Autodesk Inventor part; units mm, degrees
ref_plane "YZ Plane" through (0, 0, 0) normal (1, 0, 0) x (0, 1, 0)
ref_plane "XZ Plane" through (0, 0, 0) normal (0, 1, 0) x (-1, 0, 0)
ref_plane "XY Plane" through (0, 0, 0) normal (0, 0, 1) x (1, 0, 0)
sketch "Sketch1" plane through (0, 0, 0) normal (0, 1, 0) x (-1, 0, 0)
  line L0 (-25, -25) -> (25, -25)
  line L1 (25, -25) -> (25, 25)
  line L2 (25, 25) -> (-25, 25)
  line L3 (-25, 25) -> (-25, -25)
  line L4 (-25, -25) -> (25, 25) construction
  line L5 (25, -25) -> (-25, 25) construction
  point P0 (0, 0)
  dimension "d0" = 50
  dimension "d1" = 50
extrude "Extrusion1" add sketch "Sketch1" along normal blind 50
shell "Shell1" thickness 2 removed faces 0
fillet "Fillet1" radius 2 12 edges at (0, 50, 25) (-25, 25, -25) (25, 50, 0) (0, 50, -25) (-25, 50, 0) (25, 25, 25) (-25, 25, 25) (25, 25, -25) (25, 0, 0) (0, 0, 25) (0, 0, -25) (-25, 0, 0)
properties part number "block"
Read the model definition and answer for the solid it produces. Units are mm, in the model's axes. A direction names the side the tool comes from. Coordinates: 2 decimals unless noted, no trailing zeros. Order: outer loops, then holes, each group sorted by start corner. A loop starts at its lowest first (then second) coordinate and runs counter-clockwise, first axis right, second up. Notation, with made-up numbers: M 21.5,42.5 L 25.5,42.5 A22 ccw 25.5,64.5 Z; hole C 10,70.25 d10. An arc over 180 degrees is marked long. Put each result on its own line as item: value. Start each with the question number.
Item 1: Section B-B, the plane z = 8 is taken. Determine the outline of the cut face in (x, y), plus the area to 3 significant figures.
Item 2: Section A-A, the plane y = 17 is taken. Determine the outline of the cut face in (x, z), plus the area to 3 significant figures.
Item 3: Consider probe 1 along Z at (x, y) = (20, 15); probe 2 along Y at (x, z) = (14, 10). Determine where each line is inside the solid, lowest interval first. Write a range as [from, to].
Item 4: The mould has two halves that part along Z. Classify faces 1 (the face through (0, 25, -23)), 2 (the face through (24.43, 0.6, -0.32)), 3 (the face through (0.32, 0.6, 24.43)), 4 (the face through (0, 48, 0)): +Z half, -Z half, draft (parallel to the pull), parting line (faces both ways), or undercut.
Item 5: For faces 5 (the face through (0, 25, 23)), 6 (the face through (-25, 25, 0)), determine the directions among +Z, -Z, +X, -X, +Y, -Y from which every point of the face is accessible in a straight line to the end or side of a thin tool.
Computed:
1. outline: M -25,2 A2 ccw -23,0 L 23,0 A2 ccw 25,2 L 25,48 A2 ccw 23,50 L -23,50 A2 ccw -25,48 Z; hole M -23,2 L 23,2 L 23,48 L -23,48 Z
1. area: 381 mm2
2. outline: M -25,-23 A2 ccw -23,-25 L 23,-25 A2 ccw 25,-23 L 25,23 A2 ccw 23,25 L -23,25 A2 ccw -25,23 Z; hole M -23,-23 L 23,-23 L 23,23 L -23,23 Z
2. area: 381 mm2
3. probe 1: z = [-25, -23], [23, 25]
3. probe 2: y = [0, 2], [48, 50]
4. face 1: undercut
4. face 2: draft
4. face 3: +Z half
4. face 4: undercut
5. face 5: none
5. face 6: +Z, -Z, -X, +Y, -Y
